The listing builds one solid part. Answer for the finished solid, in the listing's coordinates (mm). A direction names the side the tool comes from. Give positions to 0.01 mm unless a question says otherwise; leave off trailing zeros. Order: outer loops, then holes, each group sorted by start corner. A loop starts at its lowest first (then second) coordinate and runs counter-clockwise, first axis right, second up. Notation, with made-up numbers: M 51.25,14.25 L 104.25,14.25 A23 ccw 104.25,30.25 Z; hole C 59.25,16 d1. An arc over 180 degrees is marked long. Answer as a JSON object with one key per item and string values. Group by question number.
Autodesk Inventor part; units mm, degrees
ref_plane "YZ Plane" through (0, 0, 0) normal (1, 0, 0) x (0, 1, 0)
ref_plane "XZ Plane" through (0, 0, 0) normal (0, 1, 0) x (-1, 0, 0)
ref_plane "XY Plane" through (0, 0, 0) normal (0, 0, 1) x (1, 0, 0)
sketch "Sketch1" plane through (0, 0, 0) normal (0, 1, 0) x (-1, 0, 0)
  line L0 (-3, 0) -> (-82, 0)
  line L1 (-85, -3) -> (-85, -53)
  line L2 (-82, -56) -> (-3, -56)
  line L3 (0, -53) -> (0, -3)
  arc A0 (-3, -56) -> (0, -53) centre (-3, -53) ccw
  arc A1 (0, -3) -> (-3, 0) centre (-3, -3) ccw
  arc A2 (-82, 0) -> (-85, -3) centre (-82, -3) ccw
  arc A3 (-85, -53) -> (-82, -56) centre (-82, -53) ccw
  circle A4 centre (-3.5, -52.5) radius 1.35
  circle A5 centre (-3.5, -3.5) radius 1.35
  circle A6 centre (-61.5, -52.5) radius 1.35
  circle A7 centre (-61.5, -3.5) radius 1.35
  point P0 (0, 0)
  point P1 (-85, -56)
  point P2 (-85, 0)
  point P3 (0, -56)
  dimension "d0" = 85
  dimension "d1" = 56
  dimension "d2" = 3
  dimension "d9" = 2.7
  dimension "d10" = 2.7
  dimension "d15" = 2.7
  dimension "d16" = 2.7
  dimension "d140" = 58
  dimension "d141" = 58
  dimension "d142" = 49
  dimension "d143" = 3.5
extrude "Extrusion1" add sketch "Sketch1" along normal blind 1.5
sketch "Sketch2" plane through (0, 1.5, 0) normal (0, 1, 0) x (1, 0, 0)
  circle A0 centre (3.5, 3.5) radius 1.35
  circle A1 centre (3.5, 3.5) radius 3
  circle A2 centre (3.5, 52.5) radius 1.35
  circle A3 centre (3.5, 52.5) radius 3
  circle A4 centre (61.5, 52.5) radius 1.35
  circle A5 centre (61.5, 52.5) radius 3
  circle A6 centre (61.5, 3.5) radius 1.35
  circle A7 centre (61.5, 3.5) radius 3
  point P0 (0, 0)
  dimension "d19" = 6
  dimension "d20" = 6
  dimension "d21" = 6
  dimension "d22" = 6
extrude "Extrusion2" cut sketch "Sketch2" against normal blind 0.001 contours A0 | A1 | A3 | A5 | A6 | A7
sketch "Sketch3" plane through (0, 1.5, 0) normal (0, 1, 0) x (1, 0, 0)
  line L0 (7.25, 55) -> (58.25, 55)
  line L1 (58.25, 55) -> (58.25, 50)
  line L2 (58.25, 50) -> (7.25, 50)
  line L3 (7.25, 50) -> (7.25, 55)
  line L4 (32.75, 55) -> (32.75, 50)
  line L5 (32.75, 52.5) -> (7.25, 52.5)
  line L6 (0, 53) -> (0, 3)
  line L7 (82, 56) -> (3, 56)
  circle A0 centre (3.5, 52.5) radius 1.35
  point P0 (0, 0)
  dimension "d25" = 51
  dimension "d26" = 5
  dimension "d28" = 25.5
  dimension "d29" = 2.5
  dimension "d30" = 3.5
  dimension "d152" = 7.25
extrude "Extrusion3" add sketch "Sketch3" along normal blind 8.75 contours L0 L4 L5 L3 | L0 L1 L2 L4 | L5 L4 L2 L3
sketch "Sketch4" plane through (0, 1.5, 0) normal (0, 1, 0) x (1, 0, 0)
  line L0 (1.95, 18.15) -> (6.05, 18.15)
  line L1 (6.05, 18.15) -> (6.05, 40.55)
  line L2 (6.05, 40.55) -> (1.95, 40.55)
  line L3 (1.95, 40.55) -> (1.95, 18.15)
  line L4 (4, 40.55) -> (4, 18.15)
  line L5 (1.95, 29.35) -> (6.05, 29.35)
  line L6 (0, 53) -> (0, 3)
  circle A0 centre (3.5, 3.5) radius 1.35
  point P0 (0, 0)
  dimension "d34" = 4.1
  dimension "d35" = 22.4
  dimension "d36" = 4
  dimension "d37" = 24.5
extrude "Extrusion4" add sketch "Sketch4" along normal blind 5.5 contours L3 L5 L4 L0 | L4 L5 L1 L0 | L3 L2 L4 L5 | L4 L2 L1 L5
sketch "Sketch5" plane through (0, 1.5, 0) normal (0, 1, 0) x (1, 0, 0)
  line L0 (7.93, 4.71) -> (15.97, 4.71)
  line L1 (15.97, 4.71) -> (15.97, -1.22)
  line L2 (15.97, -1.22) -> (7.93, -1.22)
  line L3 (7.93, -1.22) -> (7.93, 4.71)
  line L4 (3, 0) -> (82, 0)
  line L5 (11.95, -1.22) -> (11.95, 4.71)
  circle A0 centre (3.5, 3.5) radius 1.35
  point P0 (0, 0)
  dimension "d44" = 1.22
  dimension "d45" = 5.93
  dimension "d46" = 8.04
  dimension "d74" = 7.1
extrude "Extrusion5" add sketch "Sketch5" along normal blind 3.2 contours L0 L5 L4 L3 | L0 L1 L4 L5 | L4 L5 L2 L3 | L4 L1 L2 L5
sketch "Sketch6" plane through (0, 1.5, 0) normal (0, 1, 0) x (1, 0, 0)
  line L0 (7.93, -1.22) -> (15.97, -1.22)
  line L1 (11.95, -1.22) -> (11.95, 4.71)
  line L2 (7.93, 4.71) -> (15.97, 4.71)
  line L3 (24.75, 10.65) -> (39.25, 10.65)
  line L4 (39.25, 10.65) -> (39.25, -1.5)
  line L5 (39.25, -1.5) -> (24.75, -1.5)
  line L6 (24.75, -1.5) -> (24.75, 10.65)
  line L7 (15.97, 0) -> (82, 0)
  circle A0 centre (3.5, 3.5) radius 1.35
  line L8 (0, 53) -> (0, 3)
  point P0 (0, 0)
  dimension "d144" = 14.5
  dimension "d145" = 12.15
  dimension "d146" = 1.5
  dimension "d153" = 24.75
extrude "Extrusion6" add sketch "Sketch6" along normal blind 6.5 contours L3 L4 L7 L6 | L7 L4 L5 L6
sketch "Sketch7" plane through (0, 1.5, 0) normal (0, 1, 0) x (1, 0, 0)
  line L0 (1.95, 40.55) -> (1.95, 18.15)
  line L1 (6.05, 18.15) -> (6.05, 40.55)
  line L2 (42.95, 22.7) -> (47.05, 22.7)
  line L3 (47.05, 22.7) -> (47.05, 0.3)
  line L4 (47.05, 0.3) -> (42.95, 0.3)
  line L5 (42.95, 0.3) -> (42.95, 22.7)
  line L6 (45, 0.3) -> (45, 22.7)
  line L7 (42.95, 11.5) -> (47.05, 11.5)
  line L8 (0, 53) -> (0, 3)
  point P0 (0, 0)
  dimension "d78" = 4.1
  dimension "d80" = 22.4
  dimension "d150" = 45
extrude "Extrusion7" add sketch "Sketch7" along normal blind 5.5
sketch "Sketch8" plane through (0, 1.5, 0) normal (0, 1, 0) x (1, 0, 0)
  line L0 (50, 0) -> (57, 0)
  line L1 (57, 0) -> (57, 12.5)
  line L2 (57, 12.5) -> (50, 12.5)
  line L3 (50, 12.5) -> (50, 0)
  line L4 (50, 6.25) -> (57, 6.25)
  line L5 (53.5, 0) -> (53.5, 12.5)
  line L6 (3, 0) -> (82, 0)
  line L7 (47.05, 0.3) -> (42.95, 0.3)
  line L8 (45, 0.3) -> (45, 22.7)
  line L9 (42.95, 22.7) -> (47.05, 22.7)
  circle A0 centre (3.5, 3.5) radius 1.35
  line L10 (0, 53) -> (0, 3)
  point P0 (0, 0)
  point P1 (43.35, 0)
  dimension "d85" = 7
  dimension "d86" = 12.5
  dimension "d89" = 0
  dimension "d149" = 53.5
extrude "Extrusion8" add sketch "Sketch8" along normal blind 6 contours L3 L4 L5 L0 | L5 L4 L1 L0 | L3 L2 L5 L4 | L5 L2 L1 L4
sketch "Sketch9" plane through (3, 0, 0) normal (0, 0, 1) x (1, 0, 0)
  line L0 (54, 7.5) -> (47, 7.5)
  line L1 (54, 1.5) -> (54, 7.5)
  circle A0 centre (50.5, 4.25) radius 3
  point P0 (-3, 0)
  dimension "d96" = 3.5
  dimension "d97" = 3.25
  dimension "d98" = 6
extrude "Extrusion9" add sketch "Sketch9" along normal blind 2.5
sketch "Sketch10" plane through (0, 1.5, 0) normal (0, 1, 0) x (1, 0, 0)
  line L0 (66.65, 18) -> (88, 18)
  line L1 (88, 18) -> (88, 2.5)
  line L2 (88, 2.5) -> (66.65, 2.5)
  line L3 (66.65, 2.5) -> (66.65, 18)
  line L4 (85, 3) -> (85, 53)
  line L5 (88, 10.25) -> (66.65, 10.25)
  line L6 (57, 0) -> (82, 0)
  point P0 (0, 0)
  dimension "d101" = 21.35
  dimension "d102" = 15.5
  dimension "d103" = 3
  dimension "d104" = 10.25
extrude "Extrusion10" add sketch "Sketch10" along normal blind 13.5
sketch "Sketch11" plane through (0, 1.5, 0) normal (0, 1, 0) x (1, 0, 0)
  line L0 (70.3341, 22.43) -> (87.5, 22.43)
  line L1 (88, 2.4833) -> (88, 15.6315)
  line L2 (87.5, 35.57) -> (70.3341, 35.57)
  line L3 (70.3341, 35.57) -> (70.3341, 22.43)
  line L4 (85, 3) -> (85, 53)
  line L5 (88, 36.35) -> (87.5, 36.35)
  line L6 (87.5, 21.65) -> (88, 21.65)
  line L7 (88, 21.65) -> (88, 36.35)
  line L8 (87.5, 36.35) -> (87.5, 35.57)
  line L9 (87.5, 22.43) -> (87.5, 21.65)
  line L10 (88, 29) -> (70.3341, 29)
  line L11 (70.3, 40.43) -> (87.5, 40.43)
  line L12 (88, 22.6143) -> (88, 34.7304)
  line L13 (87.5, 53.57) -> (70.3, 53.57)
  line L14 (70.3, 53.57) -> (70.3, 40.43)
  line L15 (88, 54.35) -> (87.5, 54.35)
  line L16 (87.5, 39.65) -> (88, 39.65)
  line L17 (88, 39.65) -> (88, 54.35)
  line L18 (87.5, 54.35) -> (87.5, 53.57)
  line L19 (87.5, 40.43) -> (87.5, 39.65)
  line L20 (88, 47) -> (70.3, 47)
  line L21 (66.65, 2.5) -> (66.65, 18)
  line L22 (66.65, 10.25) -> (88, 10.25)
  line L23 (57, 0) -> (82, 0)
  point P0 (0, 0)
  point P1 (85, 38)
  point P2 (88, 34.35)
  dimension "d107" = 3
  dimension "d109" = 13.14
  dimension "d113" = 14.7
  dimension "d115" = 13.14
  dimension "d119" = 14.7
  dimension "d123" = 29
  dimension "d125" = 14.7
  dimension "d126" = 3
  dimension "d127" = 3
  dimension "d129" = 2.5
  dimension "d130" = 2.5
  dimension "d131" = 2.5
  dimension "d132" = 14.6659
  dimension "d133" = 3
  dimension "d134" = 34.7304
  dimension "d135" = 22.6143
  dimension "d136" = 15.6315
  dimension "d137" = 2.4833
  dimension "d151" = 47
extrude "Extrusion11" add sketch "Sketch11" along normal blind 16
properties part number "RaspberryPi3B_Mockup"
Item 1: Section D-D (x = 52) is taken. Determine the outline of the cut face in (y, z), and give its area (3 significant figures).
Item 2: Determine the mould class of faces 4 (the flat face through (88, 9, -29)), 5 (the flat face through (70.3, 9, -47)), 6 (the flat face through (7.25, 6, -52)), 7 (the flat face through (32, 5, 1.5)) for opening direction X: released by +X, released by -X, zero draft, split by the parting line, or undercut.
Item 3: Section A-A (y = 12.25) is taken. Determine the outline of the cut face in (x, z), and give its area (3 significant figures).
Item 4: Section B-B (x = 61.5) is taken. Count the separate pieces of the cut face and the enclosed holes in it, and give its area (3 significant figures).
Item 5: A tool of negligible diameter and unlimited length cuts with its end or side. For faces 1 (the flat face through (53, 7.5, -6)), 2 (the flat face through (7.93, 3, -2)), 3 (the flat face through (79, 9, -22.43)), from which of +Z, -Z, +X, -X, +Y, -Y can it reach the whole face along a straight path? Write none if from no direction.
Item 6: Consider probe 1 along Z at (x, y) = (61.5, 0.4); probe 2 along X at (y, z) = (0.45, -3.5); probe 3 along X at (y, z) = (3.5, -13). Determine where each line is inside the solid, lowest interval first. Write a range as from..to.
Item 7: Section C-C (z = -43) is taken. Determine the outline of the cut face in (x, y), and give its area (3 significant figures).
Item 8: Flat-ended cylindrical pins translate along their axes: P1, Ø5, axis at x = 60.5, z = -53.5, coming from the +Y side; P2, Ø4, axis at y = 6, z = -31, coming from the -X side; P3, Ø3.5, axis at x = 35.5, z = -7.5, coming from the +Y side. Find the tip coordinate at first contact, or state that the pin passes through.
Values found:
{
 "1": {"outline": "M 0,-56 L 1.5,-56 L 1.5,-55 L 10.25,-55 L 10.25,-50 L 1.5,-50 L 1.5,-12.5 L 7.5,-12.5 L 7.5,0 L 6.85,0 L 6.85,2.5 L 1.65,2.5 L 1.65,0 L 0,0 Z", "area": "216 mm^2"},
 "2": {"face 4": "released by +X", "face 5": "undercut", "face 6": "released by -X", "face 7": "zero draft"},
 "3": {"outline": "M 66.65,-18 L 88,-18 L 88,-2.5 L 66.65,-2.5 Z; M 70.3,-53.57 L 87.5,-53.57 L 87.5,-54.35 L 88,-54.35 L 88,-39.65 L 87.5,-39.65 L 87.5,-40.43 L 70.3,-40.43 Z; M 70.33,-35.57 L 87.5,-35.57 L 87.5,-36.35 L 88,-36.35 L 88,-21.65 L 87.5,-21.65 L 87.5,-22.43 L 70.33,-22.43 Z", "area": "797 mm^2"},
 "4": {"separate pieces": "3", "enclosed holes": "0", "area": "75.9 mm^2"},
 "5": {"face 1": "+Z, +Y", "face 2": "+Z, -X, +Y", "face 3": "+Y"},
 "6": {"probe 1": "z = -56..-53.85, -51.15..-4.85, -2.15..0", "probe 2": "x = 0..2.15, 4.85..60.15, 62.85..85", "probe 3": "x = 42.95..47.05, 66.65..88"},
 "7": {"outline": "M 0,0 L 85,0 L 85,1.5 L 88,1.5 L 88,17.5 L 70.3,17.5 L 70.3,1.5 L 0,1.5 Z", "area": "411 mm^2"},
 "8": {"P1": "stops at y = 10.25", "P2": "stops at x = 1.95", "P3": "stops at y = 8"}
}
